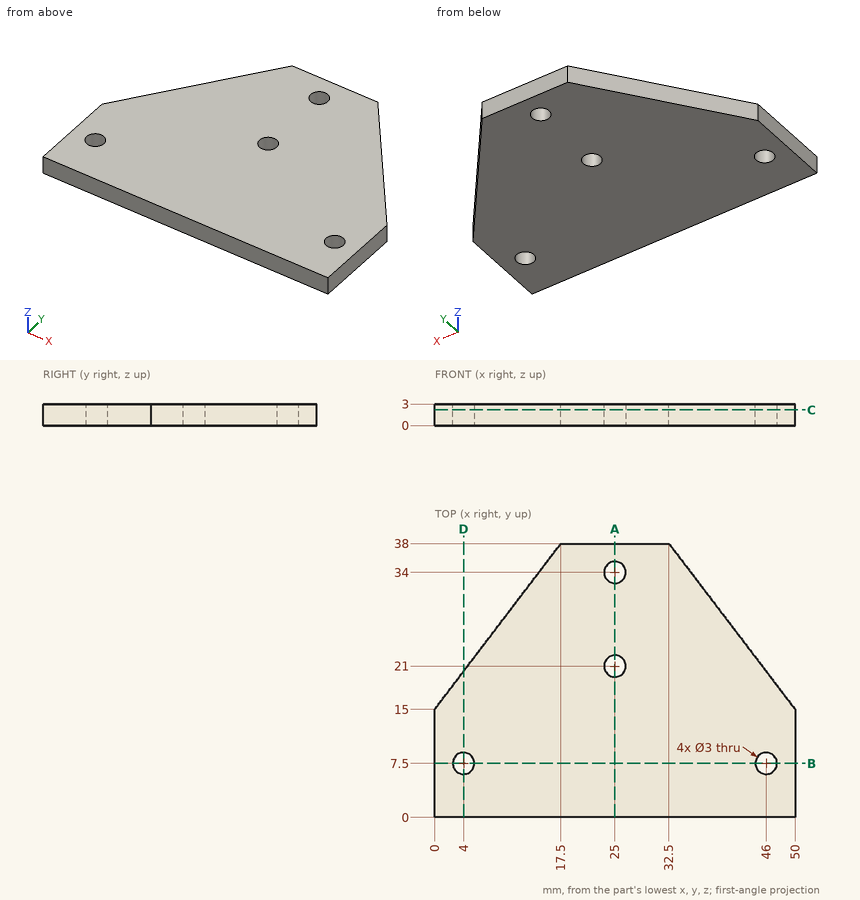
For this review, use the dimensioned drawing (mm, ordinates from the lowest corner) and the shaded views. Give positions to 0.01 mm unless a question says otherwise; leave off trailing zeros. Loops run counter-clockwise (first coordinate to the right, second up) from the corner with the lowest first, then second, coordinate; pieces in that order, holes last.
Item 1: Take a section at B-B, the plane y = 7.5. State the section outline as (x, z) points.
Item 2: Take a section at C-C, the plane z = 2.2. State the section outline as (x, y) points, and give its area (3 significant figures).
Item 3: Insertion check: pin 1 (1.8 mm diameter, centred on x = 4, y = 7.5, fed in from +Z). The pin has a flat end and moves straight along its axis. Give the tip position at first contact, or say it passes through.
Item 4: Take a section at A-A, the plane x = 25. State the section outline as (y, z) points, and give its area (3 significant figures).
Item 5: Take a section at D-D, the plane x = 4. State the section outline as (y, z) points.
Item 6: For line 1 along Y through (x, z) = (25, 1.05); line 2 along Y through (x, z) = (46, 1.45); line 3 along Y through (x, z) = (36.5, 0.5), list the stretches that pass through material, from the lowest coordinate up.
Calculated:
1. outline: (0, 0) - (2.5, 0) - (2.5, 3) - (0, 3) - close; (5.5, 0) - (44.5, 0) - (44.5, 3) - (5.5, 3) - close; (47.5, 0) - (50, 0) - (50, 3) - (47.5, 3) - close
2. outline: (0, 0) - (50, 0) - (50, 15) - (32.5, 38) - (17.5, 38) - (0, 15) - close; hole circle Ø3 at (4, 7.5); hole circle Ø3 at (25, 21); hole circle Ø3 at (25, 34); hole circle Ø3 at (46, 7.5)
2. area: 1,470 mm2
3. pin 1: passes through
4. outline: (0, 0) - (19.5, 0) - (19.5, 3) - (0, 3) - close; (22.5, 0) - (32.5, 0) - (32.5, 3) - (22.5, 3) - close; (35.5, 0) - (38, 0) - (38, 3) - (35.5, 3) - close
4. area: 96.0 mm2
5. outline: (0, 0) - (6, 0) - (6, 3) - (0, 3) - close; (9, 0) - (20.26, 0) - (20.26, 3) - (9, 3) - close
6. line 1: y = 0 to 19.5, 22.5 to 32.5, 35.5 to 38
6. line 2: y = 0 to 6, 9 to 20.26
6. line 3: y = 0 to 32.74
